```python
from build123d import *

# Parameters (mm, degrees)
BOSS_EXTRUDE1_DEPTH = 12.35
BOSS_EXTRUDE2_DEPTH = 4.3
SKETCH3_R           = 2.4
BOSS_EXTRUDE3_DEPTH = 3.25
SKETCH4_W           = 8.2
SKETCH4_H           = 3
BOSS_EXTRUDE4_DEPTH = 3
CUT_EXTRUDE1_DEPTH  = 3


with BuildPart() as part:
    # Sketch1 → Boss-Extrude1 (new body)
    with BuildSketch(Plane.XY):
        Polygon((0, 0), (22.5, 0), (22.5, 15.6), (27.5, 15.6), (27.5, 18.1), (22.5, 18.1), (22.5, 22.3), (0, 22.3), (0, 18.1), (-5, 18.1), (-5, 15.6), (0, 15.6), align=None)
    extrude(amount=BOSS_EXTRUDE1_DEPTH)

    # Sketch2 → Boss-Extrude2 (add)
    with BuildSketch(Plane(origin=(0, 22.3, 0), x_dir=(1, 0, 0), z_dir=(0, 1, 0))):
        with BuildLine():
            ThreePointArc((10.897447917, -9.119877482), (22.5, -6.175), (10.897447917, -3.230122518))
            ThreePointArc((10.897447917, -3.230122518), (7.325, -6.175), (10.897447917, -9.119877482))
        make_face()
    extrude(amount=BOSS_EXTRUDE2_DEPTH)

    # Sketch3 → Boss-Extrude3 (add)
    with BuildSketch(Plane(origin=(0, 26.6, 0), x_dir=(1, 0, 0), z_dir=(0, 1, 0))):
        with Locations((16.325, -6.175)):
            Circle(SKETCH3_R)
    extrude(amount=BOSS_EXTRUDE3_DEPTH)

    # Sketch4 → Boss-Extrude4 (add)
    with BuildSketch(Plane(origin=(22.5, 0, 0), x_dir=(0, 0, -1), z_dir=(1, 0, 0))):
        with Locations((-6.175, 5.8)):
            Rectangle(SKETCH4_W, SKETCH4_H)
    extrude(amount=BOSS_EXTRUDE4_DEPTH)

    # Sketch5 → Cut-Extrude1 (cut)
    with BuildSketch(Plane(origin=(0, 18.1, 0), x_dir=(1, 0, 0), z_dir=(0, 1, 0))):
        with BuildLine():
            Line((-3.421954446, -5.575), (-5, -5.575))
            Line((-5, -5.575), (-5, -6.775))
            Line((-5, -6.775), (-3.421954446, -6.775))
            ThreePointArc((-3.421954446, -6.775), (-1.4, -6.175), (-3.421954446, -5.575))
        make_face()
        with BuildLine():
            Line((25.921954446, -6.775), (27.5, -6.775))
            Line((27.5, -6.775), (27.5, -5.575))
            Line((27.5, -5.575), (25.921954446, -5.575))
            ThreePointArc((25.921954446, -5.575), (23.9, -6.175), (25.921954446, -6.775))
        make_face()
    extrude(amount=-CUT_EXTRUDE1_DEPTH, mode=Mode.SUBTRACT)


solid = part.part
```
Design review of the part built by this model. Coordinates are the model's own, in mm. A direction names the side the tool comes from. Round coordinates to 2 decimals unless told otherwise and drop trailing zeros. Order: outer loops, then holes, each group sorted by start corner. A loop starts at its lowest first (then second) coordinate and runs counter-clockwise, first axis right, second up. Notation, with made-up numbers: (39.25, -11.5) - (81.25, -11.5) arc R11 cw to (81.25, -1.5) - close; hole circle Ø8 at (7, 83.5). An arc over 180 degrees is marked (long way). Return JSON: item names as keys, results as strings.
Q1. Consider section C-C on y = 5.5. Write out the cut boundary in (x, z) (3 decimals).
Computed values:
{"outline": "(0, 0) - (22.5, 0) - (22.5, 2.075) - (25.5, 2.075) - (25.5, 10.275) - (22.5, 10.275) - (22.5, 12.35) - (0, 12.35) - close"}
Q2. Wall thickness on L1, parallel to Y at x = 24, z = 5.5; L2, parallel to Z at x = 25, y = 16.55 (3 decimals); L3, parallel to X at y = 21, z = 8.25: over which ranges is each line inside the solid? List them lowest first. Write a range as [from, to].
Computed values:
{"L1": "y = [4.3, 7.3], [15.6, 18.1]", "L2": "z = [0, 5.075], [7.275, 12.35]", "L3": "x = [0, 22.5]"}
Q3. For pin 1 Ø2.5 at (x, z) = (-2, 8) entering from -Y; pin 2 Ø1.5 at (y, z) = (25, 7) entering from +X; pin 3 Ø3 at (x, y) = (18, 26.5) entering from +Z, all flat-tipped, find the tip position at first contact; note any pin that passes through.
Computed values:
{"pin 1": "stops at y = 15.6", "pin 2": "stops at x = 22.5", "pin 3": "stops at z = 12.35"}
Q4. Consider section B-B on x = 25. Write out the cut boundary in (y, z) (3 decimals), plus the area to 3 significant figures.
Computed values:
{"outline": "(4.3, 2.075) - (7.3, 2.075) - (7.3, 10.275) - (4.3, 10.275) - close; (15.6, 0) - (18.1, 0) - (18.1, 5.075) - (15.6, 5.075) - close; (15.6, 7.275) - (18.1, 7.275) - (18.1, 12.35) - (15.6, 12.35) - close", "area": "50.0 mm2"}
Q5. Machinability: for faces 4 (the flat face through (-4, 17, 5.575)), 5 (the flat face through (21, 22.3, 1)), 6 (the flat face through (0, 8, 6)), which of the approach directions +Z, -Z, +X, -X, +Y, -Y give a long, thin tool a straight path to every point of the face, cutting with its end or side? Answer none if there is none.
Computed values:
{"face 4": "-X, +Y, -Y", "face 5": "-Z, +X, +Y", "face 6": "+Z, -Z, -X, -Y"}
Q6. Consider section A-A on x = -2.5. Write out the cut boundary in (y, z) (3 decimals).
Computed values:
{"outline": "(15.6, 0) - (18.1, 0) - (18.1, 5.075) - (15.6, 5.075) - close; (15.6, 7.275) - (18.1, 7.275) - (18.1, 12.35) - (15.6, 12.35) - close"}
Q7. The part is to be moulded in two halves that separate along Y. For faces 1 (the flat face through (25, 18.1, 4.7)), 2 (the flat face through (24, 4.3, 6)), 3 (the flat face through (25, 15.6, 4.7)), say which applies: pulls with the +Y half, pulls with the -Y half, needs draft (parallel to the pull), parting line crosses it, or undercut.
Computed values:
{"face 1": "pulls with the +Y half", "face 2": "pulls with the -Y half", "face 3": "undercut"}
Q8. Consider section D-D on z = 8. Write out the cut boundary in (x, y).
Computed values:
{"outline": "(-5, 15.6) - (0, 15.6) - (0, 0) - (22.5, 0) - (22.5, 4.3) - (25.5, 4.3) - (25.5, 7.3) - (22.5, 7.3) - (22.5, 15.6) - (27.5, 15.6) - (27.5, 18.1) - (22.5, 18.1) - (22.5, 22.3) - (22.22, 22.3) - (22.22, 26.6) - (17.88, 26.6) - (17.88, 29.85) - (14.77, 29.85) - (14.77, 26.6) - (7.94, 26.6) - (7.94, 22.3) - (0, 22.3) - (0, 18.1) - (-5, 18.1) - close"}
